Autodesk Inventor part; units mm, degrees
ref_plane "YZ Plane" through (0, 0, 0) normal (1, 0, 0) x (0, 1, 0)
ref_plane "XZ Plane" through (0, 0, 0) normal (0, 1, 0) x (-1, 0, 0)
ref_plane "XY Plane" through (0, 0, 0) normal (0, 0, 1) x (1, 0, 0)
sketch "Sketch1" plane through (0, 0, 0) normal (0, 1, 0) x (-1, 0, 0)
  line L0 (-9.2268, 12.0612) -> (9.2268, 12.0612)
  line L1 (9.2268, -12.0612) -> (-9.2268, -12.0612)
  line L2 (-9.2268, -12.0612) -> (-9.2268, 12.0612)
  line L3 (-9.2268, 12.0612) -> (9.2268, -12.0612) construction
  line L4 (9.2268, 12.0612) -> (-9.2268, -12.0612) construction
  line L5 (-4.2415, 4.8647) -> (9.2268, 4.8647)
  line L6 (9.2268, -4.8647) -> (-4.2415, -4.8647)
  line L7 (-4.2415, -4.8647) -> (-4.2415, 4.8647)
  line L8 (-4.2415, 4.8647) -> (14.8956, -4.8647) construction
  line L9 (14.8956, 4.8647) -> (-4.2415, -4.8647) construction
  line L10 (9.2268, 12.0612) -> (9.2268, 4.8647)
  line L11 (9.2268, -4.8647) -> (9.2268, -12.0612)
  point P0 (0, 0)
  point P1 (5.327, 0)
extrude "Extrusion1" add sketch "Sketch1" along normal blind 20
properties part number "slot"
Input: part model. Units: mm. Frame: model coordinates. A direction names the side the tool comes from. Coordinates: 2 decimals unless noted, no trailing zeros. Loops run counter-clockwise (first coordinate to the right, second up) from the corner with the lowest first, then second, coordinate; pieces in that order, holes last. Notation, with made-up numbers: (85, 77.5) -> (114, 77.5) arc R27 cw to (114, 103.5) -> close; hole circle Ø4 at (70.25, -8). An arc over 180 degrees is marked (long way). Write each question's results on one line, items separated by ' | '. Start each with the question number.
Q1. Pin query (flat end, axial travel): pin 1 (6 mm diameter, centred on x = -2.5, z = 1, fed in from -Y). Return the tip coordinate at first contact, or that it passes through.
Q2. Reachability of faces 5 (the flat face through (-9.227, 10, 9)), 6 (the flat face through (-3, 10, -4.865)) from +Z, -Z, +X, -X, +Y, -Y: full face, straight path, thin tool, end or side. Return the list, or none.
Q3. Pull-direction query (Z, two-part tool) for faces 1 (the flat face through (0, 10, -12.061)), 2 (the flat face through (9.227, 10, 0)), 3 (the flat face through (4.242, 10, 0)), 4 (the flat face through (0, 10, 12.061)); classes: released by +Z, released by -Z, zero draft, split by the parting line, or undercut.
Q4. Section A-A, the plane x = 2.75. Return the cut outline in (y, z), plus the area to 3 significant figures.
Q5. Section C-C, the plane z = 1.25. Return the cut outline in (x, y).
Q6. Section B-B, the plane y = 11.5. Return the cut outline in (x, z), plus the area to 3 significant figures.
Q7. Ray query, line 1 (Z direction, x = 0.5, y = 17.75); line 2 (X direction, y = 1.5, z = -2). Return the intervals inside material, ascending. Write a range as from..to.
Found:
1) pin 1: through
2) face 5: +Z, -Z, -X, +Y, -Y | face 6: -X, +Y, -Y
3) face 1: released by -Z | face 2: zero draft | face 3: undercut | face 4: released by +Z
4) outline: (0, -12.06) -> (20, -12.06) -> (20, -4.86) -> (0, -4.86) -> close; (0, 4.86) -> (20, 4.86) -> (20, 12.06) -> (0, 12.06) -> close | area: 288 mm2
5) outline: (4.24, 0) -> (9.23, 0) -> (9.23, 20) -> (4.24, 20) -> close
6) outline: (-9.23, -12.06) -> (9.23, -12.06) -> (9.23, 12.06) -> (-9.23, 12.06) -> (-9.23, 4.86) -> (4.24, 4.86) -> (4.24, -4.86) -> (-9.23, -4.86) -> close | area: 314 mm2
7) line 1: -12.06..-4.86, 4.86..12.06 | line 2: 4.24..9.23
